Build history of the part. All positions in model axes, mm. A direction names the side the tool comes from. Round coordinates to 2 decimals unless told otherwise and drop trailing zeros. Order: outer loops, then holes, each group sorted by start corner. A loop starts at its lowest first (then second) coordinate and runs counter-clockwise, first axis right, second up. Notation, with made-up numbers: (4.25, -30.5) -> (16.25, -30.5) arc R19 cw to (16.25, -23.5) -> close; hole circle Ø7 at (-16.5, -24.75). An arc over 180 degrees is marked (long way). Write item = value, one per line.
from build123d import *

# Parameters (mm, degrees)
BOSS_EXTRUDE1_DEPTH = 160


with BuildPart() as part:
    # Sketch1 → Boss-Extrude1 (new body, symmetric)
    with BuildSketch(Plane.XY):
        Polygon((-6, -17.060660172), (-2.939339828, -14), (2.939339828, -14), (6, -17.060660172), (6, -18), (3, -18), (3, -20), (10, -20), (10, -13), (8, -13), (8, -16), (7.060660172, -16), (4, -12.939339828), (4, -7.060660172), (7.060660172, -4), (8, -4), (8, -7), (10, -7), (10, 7), (8, 7), (8, 4), (7.060660172, 4), (4, 7.060660172), (4, 12.939339828), (7.060660172, 16), (8, 16), (8, 13), (10, 13), (10, 20), (3, 20), (3, 18), (6, 18), (6, 17.060660172), (2.939339828, 14), (-2.939339828, 14), (-6, 17.060660172), (-6, 18), (-3, 18), (-3, 20), (-10, 20), (-10, 13), (-8, 13), (-8, 16), (-7.060660172, 16), (-4, 12.939339828), (-4, 7.060660172), (-7.060660172, 4), (-8, 4), (-8, 7), (-10, 7), (-10, -7), (-8, -7), (-8, -4), (-7.060660172, -4), (-4, -7.060660172), (-4, -12.939339828), (-7.060660172, -16), (-8, -16), (-8, -13), (-10, -13), (-10, -20), (-3, -20), (-3, -18), (-6, -18), align=None)
        Polygon((-6.939339828, -2), (-8, -2), (-8, 2), (-6.939339828, 2), (-2.939339828, 6), (2.939339828, 6), (6.939339828, 2), (8, 2), (8, -2), (6.939339828, -2), (2.939339828, -6), (-2.939339828, -6), align=None, mode=Mode.SUBTRACT)
    extrude(amount=BOSS_EXTRUDE1_DEPTH, both=True)


solid = part.part
Q1. Cut at A-A, the plane y = -10. List the corners of the cut face in (x, z), and give its area (3 significant figures).
Check values:
outline = (-4, -160) -> (4, -160) -> (4, 160) -> (-4, 160) -> close
area = 2,560 mm²
Q2. Probe probe 1 along Y at (x, z) = (8.5, 90); probe 2 along Y at (x, z) = (-5, 119.5); probe 3 along Y at (x, z) = (-1.75, -19). List the from-to ranges inside material, lowest first.
Check values:
probe_1 = -20 to -13, -7 to 7, 13 to 20
probe_2 = -20 to -18, -16.06 to -13.94, -6.06 to -3.94, 3.94 to 6.06, 13.94 to 16.06, 18 to 20
probe_3 = -14 to -6, 6 to 14
Q3. Which spindle directions (+Z, -Z, +X, -X, +Y, -Y) get a long thin tool onto all of the face, cutting with end or side? Do faces 4 (the face through (0, 14, 2)), 5 (the face through (4, -10, 2)), 6 (the face through (-4, 10, 2)), 7 (the face through (6, -20, 2)), 8 (the face through (0, -6, 2)). Say none if no direction does.
Check values:
face_4 = +Z, -Z, +Y
face_5 = +Z, -Z, +X
face_6 = +Z, -Z, -X
face_7 = +Z, -Z, +X, -X, -Y
face_8 = +Z, -Z
Q4. Flat gauge pin, fed straight in: pin 1 (3 mm diameter, centred on x = -0.5, z = 11, fed in from +Y). Where does the tip first touch, or does it go through?
Check values:
pin_1 = 14
Q5. Mould opens along X. For faces 1 (the face through (0, -14, 2)), 2 (the face through (-7, -20, 2)), 3 (the face through (-10, -16, 2)) say: released by +X, released by -X, zero draft, split by the parting line, or undercut.
Check values:
face_1 = undercut
face_2 = zero draft
face_3 = released by -X
